```python
from build123d import *

# Parameters (mm, degrees)
SKETCH1_R           = 12.5
BOSS_EXTRUDE1_DEPTH = 55.8
SKETCH2_R           = 1.25
CUT_EXTRUDE1_DEPTH  = 5
SKETCH2_3_R         = 3.5
BOSS_EXTRUDE2_DEPTH = 2.5
BOSS_EXTRUDE3_DEPTH = 9


with BuildPart() as part:
    # Sketch1 → Boss-Extrude1 (new body)
    with BuildSketch(Plane(origin=(0, 0, 0), x_dir=(1, 0, 0), z_dir=(0, 1, 0))):
        Circle(SKETCH1_R)
    extrude(amount=BOSS_EXTRUDE1_DEPTH)

    # Sketch2 → Cut-Extrude1 (cut)
    with BuildSketch(Plane(origin=(0, 55.8, 0), x_dir=(1, 0, 0), z_dir=(0, 1, 0))):
        with Locations((0, 10.5)):
            Circle(SKETCH2_R)
        with Locations((0, -10.5)):
            Circle(SKETCH2_R)
    extrude(amount=-CUT_EXTRUDE1_DEPTH, mode=Mode.SUBTRACT)

    # Sketch2<3> → Boss-Extrude2 (add)
    with BuildSketch(Plane(origin=(0, 55.8, 0), x_dir=(1, 0, 0), z_dir=(0, 1, 0))):
        Circle(SKETCH2_3_R)
    extrude(amount=BOSS_EXTRUDE2_DEPTH)

    # Sketch3 → Boss-Extrude3 (add)
    with BuildSketch(Plane(origin=(0, 58.3, 0), x_dir=(1, 0, 0), z_dir=(0, 1, 0))):
        with BuildLine():
            Line((1.322875656, 1.5), (-1.322875656, 1.5))
            ThreePointArc((-1.322875656, 1.5), (-0.822875656, -1.822875656), (2, 0))
            ThreePointArc((2, 0), (1.822875656, 0.822875656), (1.322875656, 1.5))
        make_face()
    extrude(amount=BOSS_EXTRUDE3_DEPTH)


solid = part.part
```
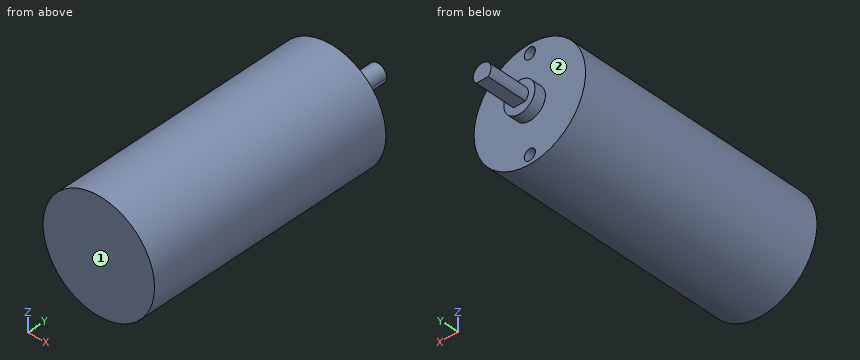
For this review, take the finished solid that the model builds, in its own axes (mm). Face numbers are marked on the shaded views. A direction names the side the tool comes from. Round coordinates to 2 decimals unless told otherwise and drop trailing zeros. Loops run counter-clockwise (first coordinate to the right, second up) from the corner with the lowest first, then second, coordinate; pieces in that order, holes last.
Q1. Add section C-C on y = 7.5. Write out the cut boundary in (x, z).
Result sheet:
outline: circle Ø25 at (0, 0)
Q2. Insertion check: pin 1 Ø10 at (x, z) = (-5, 6.5) entering from +Y; pin 2 Ø1.5 at (x, y) = (-0.5, 12.5) entering from -Z; pin 3 Ø8 at (y, z) = (56, 7) entering from +X; pin 4 Ø2 at (x, z) = (0, -10.5) entering from +Y. Each pin has a flat end and moves straight along its axis. Give the tip position at first contact, or say it passes through.
Result sheet:
pin 1: stops at y = 58.3
pin 2: stops at z = -12.5
pin 3: stops at x = 12.13
pin 4: stops at y = 50.8
Q3. Add section D-D on z = -10.5. Write out the cut boundary in (x, y).
Result sheet:
outline: (-6.78, 0) - (6.78, 0) - (6.78, 55.8) - (1.25, 55.8) - (1.25, 50.8) - (-1.25, 50.8) - (-1.25, 55.8) - (-6.78, 55.8) - close
Q4. To check wall thickness, follow line 1 along Z through (x, y) = (0, 52.8); line 2 along Y through (x, z) = (5.25, 9); line 3 along X through (y, z) = (47, 0.5). State the ranges of each line that lie inside material, in increasing order.
Result sheet:
line 1: z = -12.5 to -11.75, -9.25 to 9.25, 11.75 to 12.5
line 2: y = 0 to 55.8
line 3: x = -12.49 to 12.49
Q5. Add section B-B on z = -0.75. Write out the cut boundary in (x, y).
Result sheet:
outline: (-12.48, 0) - (12.48, 0) - (12.48, 55.8) - (3.42, 55.8) - (3.42, 58.3) - (1.85, 58.3) - (1.85, 67.3) - (-1.85, 67.3) - (-1.85, 58.3) - (-3.42, 58.3) - (-3.42, 55.8) - (-12.48, 55.8) - close
Q6. Add section A-A on x = 0. Write out the cut boundary in (y, z).
Result sheet:
outline: (0, -12.5) - (55.8, -12.5) - (55.8, -11.75) - (50.8, -11.75) - (50.8, -9.25) - (55.8, -9.25) - (55.8, -3.5) - (58.3, -3.5) - (58.3, -1.5) - (67.3, -1.5) - (67.3, 2) - (58.3, 2) - (58.3, 3.5) - (55.8, 3.5) - (55.8, 9.25) - (50.8, 9.25) - (50.8, 11.75) - (55.8, 11.75) - (55.8, 12.5) - (0, 12.5) - close
Q7. Machinability: for the marked faces 1 and 2, which of the approach directions +Z, -Z, +X, -X, +Y, -Y give a long, thin tool a straight path to every point of the face, cutting with its end or side? Answer none if there is none.
Result sheet:
face 1: +Z, -Z, +X, -X, -Y
face 2: +Y
